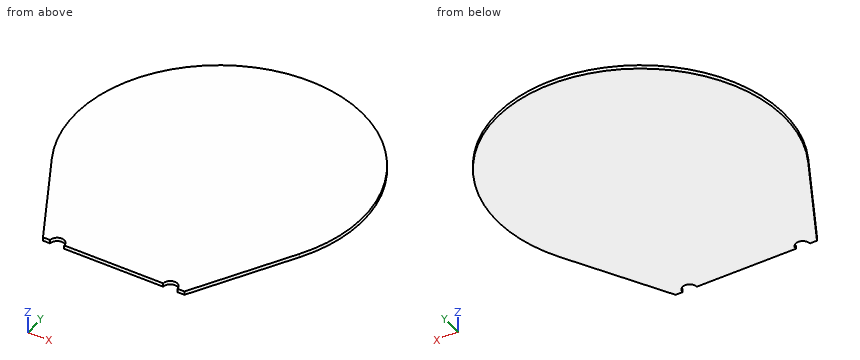
```python
from build123d import *

# Parameters (mm, degrees)
BOSS_EXTRUDE1_DEPTH   = 0.75438
CORTE_EXTRUS_O1_DEPTH = 10


with BuildPart() as part:
    # Sketch1 → Boss-Extrude1 (new body)
    with BuildSketch(Plane.XY):
        with BuildLine():
            Line((-26.292884648, -14.44590658), (-15, -35))
            Line((-15, -35), (-7.5, -35))
            Line((-7.5, -35), (15, -35))
            Line((15, -35), (26.292884648, -14.44590658))
            ThreePointArc((26.292884648, -14.44590658), (0, 30), (-26.292884648, -14.44590658))
        make_face()
    extrude(amount=BOSS_EXTRUDE1_DEPTH)

    # Esboço1 → Corte-extrusão1 (cut)
    with BuildSketch(Plane.XY.offset(0.75438)):
        with BuildLine():
            ThreePointArc((13.5, -35), (12, -33.5), (10.5, -35))
            Line((10.5, -35), (13.5, -35))
        make_face()
        with BuildLine():
            Line((13.5, -35), (10.5, -35))
            ThreePointArc((10.5, -35), (12, -36.5), (13.5, -35))
        make_face()
        with BuildLine():
            ThreePointArc((-10.5, -35), (-12, -33.5), (-13.5, -35))
            Line((-13.5, -35), (-12, -35))
            Line((-12, -35), (-10.5, -35))
        make_face()
        with BuildLine():
            Line((-12, -35), (-13.5, -35))
            ThreePointArc((-13.5, -35), (-12, -36.5), (-10.5, -35))
            Line((-10.5, -35), (-12, -35))
        make_face()
    extrude(amount=-CORTE_EXTRUS_O1_DEPTH, mode=Mode.SUBTRACT)


solid = part.part
```
Verification items for the finished model (mm, model axes). Coordinates: 2 decimals unless noted, no trailing zeros. Write each loop counter-clockwise with the first axis right and the second up, starting at its lowest first coordinate (ties: lowest second). Pieces come first, ordered by that corner, then holes. Notation, with made-up numbers: (30, 78) - (55, 78) arc R21 cw to (55, 99) - close; hole circle Ø9 at (88, -6). An arc over 180 degrees is marked (long way). One line per question, with ' | ' between items. Start each with the question number.
1. Section check C-C (x = -12). Enter the section's corners in (y, z), plus the area to 3 significant figures.
2. Section check B-B (y = -30). Enter the section's corners in (x, z), plus the area to 3 significant figures.
3. Section check A-A (z = 0.6). Enter the section's corners in (x, y), plus the area to 3 significant figures.
4. Material ranges on line 1 along X through (y, z) = (0.5, 0.7); line 2 along X through (y, z) = (14, 0.55); line 3 along Y through (x, z) = (24.5, 0.6), recorded low to high.
Computed values:
1) outline: (-33.5, 0) - (27.5, 0) - (27.5, 0.75) - (-33.5, 0.75) - close | area: 46.0 mm²
2) outline: (-17.75, 0) - (17.75, 0) - (17.75, 0.75) - (-17.75, 0.75) - close | area: 26.8 mm²
3) outline: (-26.29, -14.45) - (-15, -35) - (-13.5, -35) arc R1.5 cw to (-10.5, -35) - (10.5, -35) arc R1.5 cw to (13.5, -35) - (15, -35) - (26.29, -14.45) arc R30 ccw (long way) to start | area: 3,090 mm²
4) line 1: -30 to 30 | line 2: -26.53 to 26.53 | line 3: -17.71 to 17.31
